CAD build for the part. Positions are in the model's coordinates, mm. A direction names the side the tool comes from. Coordinates: 2 decimals unless noted, no trailing zeros. Loops run counter-clockwise (first coordinate to the right, second up) from the corner with the lowest first, then second, coordinate; pieces in that order, holes last. Notation, with made-up numbers: (-21.75, 8) -> (22.25, 8) arc R33 ccw to (22.25, 44) -> close; hole circle Ø6 at (69.25, 0). An arc over 180 degrees is marked (long way). Return JSON: item names as keys, results as strings. Group by question number.
(1) Flat gauge pins, fed straight in: pin 1 Ø8 at (y, z) = (-8, 3) entering from +X; pin 2 Ø4 at (x, z) = (-1, 13.5) entering from -Y; pin 3 Ø8 at (x, z) = (1, 2) entering from -Y. Where does each tip first touch, or does it go through?
(2) Saw through at A-A on x = 0.5. Write the cut outline in (y, z).
(3) Mould opens along X. For faces 3 (the face through (-1.62, 12.31, 13.95)), 4 (the face through (-1.936, 14.746, 13.952)), 5 (the face through (-2, 15, 12.7)) say: pulls with the +X half, pulls with the -X half, needs draft (parallel to the pull), parting line crosses it, or undercut.
(4) Saw through at B-B on y = 0. Write the cut outline in (x, z) (3 decimals).
(5) Probe L1, parallel to Y at x = 0, z = 14; L2, parallel to Z at x = -19, y = 15.5; L3, parallel to X at y = 6, z = 14.75. List the from-to ranges inside material, lowest first.
(6) Tool access for faces 1 (the face through (4.712, -15.134, 6.261)), 2 (the face through (3, -3, 12.7)): list every direction of +Z, -Z, +X, -X, +Y, -Y with a clear straight run to the whole face (end or side of a thin tool).
```python
from build123d import *

# Parameters (mm, degrees)
F0_R     = 14.8728461467
F1_DEPTH = 12.7
F2_R     = 2.54
F0_R_2   = 12.4153453857
F0_R_3   = 3.175
F3_DEPTH = 12.7
F4_DEPTH = 15.24


with BuildPart() as f1:
    # F0 (on Top) → F1 (new body)
    with BuildSketch(Plane.XY):
        with BuildLine():
            ThreePointArc((21.0967877354, -14.1451598523), (15.4923273366, -3.3399893418), (25.0509920661, 4.1961644989))
            ThreePointArc((25.0509920661, 4.1961644989), (24.1794993656, 7.778933759), (22.7984616404, 11.197774191))
            ThreePointArc((22.7984616404, 11.197774191), (10.6386792866, 11.7467543663), (8.8915109785, 23.7928777688))
            ThreePointArc((8.8915109785, 23.7928777688), (5.3529954332, 24.8295275809), (1.7016739049, 25.3429340433))
            ThreePointArc((1.7016739049, 25.3429340433), (1.7549973478, 24.7623025716), (1.7727939343, 24.1794993656))
            ThreePointArc((1.7727939343, 24.1794993656), (-5.4138971923, 14.9251974489), (-16.1594810876, 19.5967132698))
            ThreePointArc((-16.1594810876, 19.5967132698), (-18.8265039325, 17.0505938219), (-21.0967877354, 14.1451598523))
            ThreePointArc((-21.0967877354, 14.1451598523), (-16.8643026475, 10.6246833684), (-15.2777998876, 5.3529954332))
            ThreePointArc((-15.2777998876, 5.3529954332), (-18.154194875, -1.4789468377), (-25.0509920661, -4.1961644989))
            ThreePointArc((-25.0509920661, -4.1961644989), (-24.1794993656, -7.778933759), (-22.7984616404, -11.197774191))
            ThreePointArc((-22.7984616404, -11.197774191), (-12.7883506503, -10.278475793), (-7.4988661286, -18.8265039325))
            ThreePointArc((-7.4988661286, -18.8265039325), (-7.8536149844, -21.4054731432), (-8.8915109785, -23.7928777688))
            ThreePointArc((-8.8915109785, -23.7928777688), (-5.3529954332, -24.8295275809), (-1.7016739049, -25.3429340433))
            ThreePointArc((-1.7016739049, -25.3429340433), (4.8536480499, -15.0867437081), (16.1594810876, -19.5967132698))
            ThreePointArc((16.1594810876, -19.5967132698), (18.8265039325, -17.0505938219), (21.0967877354, -14.1451598523))
        make_face()
        Circle(F0_R, mode=Mode.SUBTRACT)
    extrude(amount=F1_DEPTH)

    # F2
    f2_edges = [f1.edges().sort_by_distance(p)[0] for p in [
        (1.701674, 25.342934, 6.35),
        (8.891511, 23.792878, 6.35),
        (-16.159481, 19.596713, 6.35),
        (-21.096788, 14.14516, 6.35),
        (-25.050992, -4.196164, 6.35),
        (25.050992, 4.196164, 6.35),
        (22.798462, 11.197774, 6.35),
        (21.096788, -14.14516, 6.35),
        (16.159481, -19.596713, 6.35),
        (-1.701674, -25.342934, 6.35),
        (-8.891511, -23.792878, 6.35),
        (-22.798462, -11.197774, 6.35),
    ]]
    fillet(f2_edges, radius=F2_R)



with BuildPart() as f3:
    # F0 (on Top) → F3 (new body)
    with BuildSketch(Plane.XY):
        Circle(F0_R_2)
        Circle(F0_R_3, mode=Mode.SUBTRACT)
    extrude(amount=F3_DEPTH)


with BuildPart() as f1_1:
    add(f1.part)

    add(f3.part)  # F4 merges F3
    # F0 (on Top) → F4 (join)
    with BuildSketch(Plane.XY):
        Circle(F0_R)
        Circle(F0_R_2, mode=Mode.SUBTRACT)
    extrude(amount=F4_DEPTH)


solid = f1_1.part
```
Geometry results:
{
 "1": {"pin 1": "x = 17.97", "pin 2": "y = -24.62", "pin 3": "y = -24.72"},
 "2": {"outline": "(-17.99, 0) -> (-3.14, 0) -> (-3.14, 12.7) -> (-12.41, 12.7) -> (-12.41, 15.24) -> (-14.86, 15.24) -> (-14.86, 12.7) -> (-17.99, 12.7) -> close; (3.14, 0) -> (19.42, 0) -> (19.42, 12.7) -> (14.86, 12.7) -> (14.86, 15.24) -> (12.41, 15.24) -> (12.41, 12.7) -> (3.14, 12.7) -> close"},
 "3": {"face 3": "undercut", "face 4": "parting line crosses it", "face 5": "needs draft"},
 "4": {"outline": "(-16.919, 0) -> (-3.175, 0) -> (-3.175, 12.7) -> (-12.415, 12.7) -> (-12.415, 15.24) -> (-14.873, 15.24) -> (-14.873, 12.7) -> (-16.919, 12.7) -> close; (3.175, 0) -> (16.919, 0) -> (16.919, 12.7) -> (14.873, 12.7) -> (14.873, 15.24) -> (12.415, 15.24) -> (12.415, 12.7) -> (3.175, 12.7) -> close"},
 "5": {"L1": "-14.87 to -12.42, 12.42 to 14.87", "L2": "0 to 12.7", "L3": "-13.61 to -10.87, 10.87 to 13.61"},
 "6": {"face 1": "+Z, -Z, -Y", "face 2": "+Z"}
}
